Read the model definition and answer for the solid it produces. Units are mm, in the model's axes. A direction names the side the tool comes from. Give positions to 0.01 mm unless a question says otherwise; leave off trailing zeros. Loops run counter-clockwise (first coordinate to the right, second up) from the corner with the lowest first, then second, coordinate; pieces in that order, holes last. Notation, with made-up numbers: (89.5, -23.5) -> (114.5, -23.5) arc R16 ccw to (114.5, -4.5) -> close; hole circle Ø5 at (-12.75, 79.5). An arc over 180 degrees is marked (long way). Write each question's results on one line, items separated by ' | '. Start each with the question number.
Item 1: Section B-B on y = 36 is taken. Write down the section's boundary in (x, z), and give its area (3 significant figures).
Item 2: Section C-C on z = 29 is taken. Write down the section's boundary in (x, y).
Item 3: Find the intervals of material crossed by line 1 (Z direction, x = 8.25, y = 38); line 2 (Z direction, x = 1.75, y = 14); line 3 (Z direction, x = 9, y = 20.5), in increasing order.
Item 4: Which of the six approach directions +Z, -Z, +X, -X, +Y, -Y give full straight-line access (tool end or side, diameter ignored) to faces 1 (the flat face through (10, 39, 61)), 2 (the flat face through (5, 14, 88.886)), 3 (the flat face through (10, 23, 94)), 4 (the flat face through (5, 31, 94.686)), 5 (the flat face through (6, 39.749, 39))?
Item 5: Determine the mould class of faces 6 (the flat face through (0, 38, 61)), 7 (the cylindrical face through (5.078, 13.559, 19.413)), 8 (the cylindrical face through (8.476, 37.214, 77.586)), 9 (the flat face through (5, 30, 26.686)) for opening direction Z: +Z half, -Z half, draft (parallel to the pull), parting line (faces both ways), or undercut.
Item 6: Each of these flat-tipped pins is pushed along its axis until it touches: P1, Ø2, axis at y = 29.5, z = 86.5, coming from the -X side; P2, Ø3, axis at x = 5, z = 21.19, coming from the +Y side; P3, Ø5, axis at x = 6, y = 31.5, coming from the -Z side; P4, Ø2.5, axis at y = 37.5, z = 60.5, coming from the +X side. Where does it stop, or does it pass through?
Item 7: Section D-D on z = 54.5 is taken. Write down the section's boundary in (x, y).
Item 8: Section A-A on y = 23 is taken. Write down the section's boundary in (x, z).
```python
from build123d import *

# Parameters (mm, degrees)
BOSS_EXTRUDE1_DEPTH = 10
SKETCH2_R           = 1.775
CUT_EXTRUDE1_DEPTH  = 112.599557576
SKETCH3_W           = 10
SKETCH3_H           = 8.5
BOSS_EXTRUDE2_DEPTH = 2
SKETCH4_R           = 1.775
CUT_EXTRUDE2_DEPTH  = 115.036008573
FILLET2_R           = 0.5
FILLET3_R           = 2
SKETCH5_W           = 10
SKETCH5_H           = 56.4
CUT_EXTRUDE3_DEPTH  = 10
SKETCH6_R           = 3.25
CUT_EXTRUDE4_DEPTH  = 5


with BuildPart() as part:
    # Sketch1 → Boss-Extrude1 (new body)
    with BuildSketch(Plane(origin=(0, 0, 0), x_dir=(0, 0, -1), z_dir=(1, 0, 0))):
        Polygon((-108.186003028, 9.249121329), (-86.186003028, 9.249121329), (-86.186003028, 34.749121329), (-35.186003028, 34.749121329), (-35.186003028, 9.249121329), (-13.186003028, 9.249121329), (-13.186003028, 17.749121329), (-26.686003028, 17.749121329), (-26.686003028, 43.249121329), (-94.686003028, 43.249121329), (-94.686003028, 17.749121329), (-108.186003028, 17.749121329), align=None)
    extrude(amount=BOSS_EXTRUDE1_DEPTH)

    # Sketch2 → Cut-Extrude1 (cut, through all)
    with BuildSketch(Plane(origin=(0, 17.749121329, 0), x_dir=(1, 0, 0), z_dir=(0, 1, 0))):
        with Locations(Location((5, -100.186003028, 0), (0, 0, 270))):
            Circle(SKETCH2_R)
        with Locations(Location((5, -21.186003028, 0), (0, 0, 270))):
            Circle(SKETCH2_R)
    extrude(amount=-CUT_EXTRUDE1_DEPTH, mode=Mode.SUBTRACT)

    # Sketch3 → Boss-Extrude2 (add)
    with BuildSketch(Plane(origin=(10, 0, 0), x_dir=(0, 0, -1), z_dir=(1, 0, 0))):
        with Locations((-80.686003028, 38.999121329)):
            Rectangle(SKETCH3_W, SKETCH3_H)
        with Locations((-40.686003028, 38.999121329)):
            Rectangle(SKETCH3_W, SKETCH3_H)
    extrude(amount=BOSS_EXTRUDE2_DEPTH)

    # Sketch4 → Cut-Extrude2 (cut, through all)
    with BuildSketch(Plane(origin=(0, 43.249121329, 0), x_dir=(1, 0, 0), z_dir=(0, 1, 0))):
        with Locations(Location((7.5, -80.686003028, 0), (0, 0, 270))):
            Circle(SKETCH4_R)
        with Locations(Location((7.5, -40.686003028, 0), (0, 0, 270))):
            Circle(SKETCH4_R)
    extrude(amount=-CUT_EXTRUDE2_DEPTH, mode=Mode.SUBTRACT)

    # Fillet2
    fillet2_edges = [part.edges().sort_by_distance(p)[0] for p in [
        (10, 38.999121329, 35.686003028),
        (10, 38.999121329, 45.686003028),
        (12, 38.999121329, 35.686003028),
        (12, 38.999121329, 45.686003028),
        (10, 38.999121329, 75.686003028),
        (12, 38.999121329, 75.686003028),
        (12, 38.999121329, 85.686003028),
        (10, 38.999121329, 85.686003028),
    ]]
    fillet(fillet2_edges, radius=FILLET2_R)

    # Fillet3
    fillet3_edges = [part.edges().sort_by_distance(p)[0] for p in [
        (0, 13.499121329, 13.186003028),
        (0, 13.499121329, 108.186003028),
        (10, 13.499121329, 13.186003028),
        (10, 13.499121329, 108.186003028),
    ]]
    fillet(fillet3_edges, radius=FILLET3_R)

    # Sketch5 → Cut-Extrude3 (cut)
    with BuildSketch(Plane.XZ.offset(-9.249121329)):
        with Locations((5, 60.686003028)):
            Rectangle(SKETCH5_W, SKETCH5_H)
    extrude(amount=-CUT_EXTRUDE3_DEPTH, mode=Mode.SUBTRACT)

    # Sketch6 → Cut-Extrude4 (cut)
    with BuildSketch(Plane.XZ.offset(-34.749121329)):
        with Locations(Location((7.5, 80.686003028, 0), (0, 0, 270))):
            Circle(SKETCH6_R)
        with Locations(Location((7.5, 40.686003028, 0), (0, 0, 270))):
            Circle(SKETCH6_R)
    extrude(amount=-CUT_EXTRUDE4_DEPTH, mode=Mode.SUBTRACT)


solid = part.part
```
Findings:
1) outline: (0, 26.69) -> (10, 26.69) -> (10, 35.19) arc R0.5 cw to (10.5, 35.69) -> (11.5, 35.69) arc R0.5 ccw to (12, 36.19) -> (12, 45.19) arc R0.5 ccw to (11.5, 45.69) -> (10.5, 45.69) arc R0.5 cw to (10, 46.19) -> (10, 75.19) arc R0.5 cw to (10.5, 75.69) -> (11.5, 75.69) arc R0.5 ccw to (12, 76.19) -> (12, 85.19) arc R0.5 ccw to (11.5, 85.69) -> (10.5, 85.69) arc R0.5 cw to (10, 86.19) -> (10, 94.69) -> (0, 94.69) -> close; hole circle Ø6.5 at (7.5, 40.69); hole circle Ø6.5 at (7.5, 80.69) | area: 654 mm2
2) outline: (0, 9.25) -> (10, 9.25) -> (10, 43.25) -> (0, 43.25) -> close
3) line 1: 26.69 to 37.52, 43.85 to 77.52, 83.85 to 94.69 | line 2: 13.2 to 32.49, 88.89 to 108.17 | line 3: 26.69 to 35.19, 86.19 to 94.69
4) face 1: +X, +Y, -Y | face 2: +X, -X, -Y | face 3: +Z, +X, +Y, -Y | face 4: +Z, +X, -X, +Y | face 5: -Y
5) face 6: draft | face 7: undercut | face 8: undercut | face 9: -Z half
6) P1: x = 0 | P2: through | P3: z = 26.69 | P4: x = 10
7) outline: (0, 34.75) -> (10, 34.75) -> (10, 43.25) -> (0, 43.25) -> close
8) outline: (0, 26.69) -> (10, 26.69) -> (10, 35.19) -> (0, 35.19) -> close; (0, 86.19) -> (10, 86.19) -> (10, 94.69) -> (0, 94.69) -> close
